Part model, mm, in its own coordinate system. Give positions to 0.01 mm unless a question says otherwise; leave off trailing zeros. Write each loop counter-clockwise with the first axis right and the second up, starting at its lowest first coordinate (ties: lowest second). Pieces come first, ordered by that corner, then holes. Notation, with made-up numbers: (-27.75, -7.5) - (-11.75, -7.5) arc R26 ccw to (-11.75, 10.5) - close; hole circle Ø4 at (53.25, 64.5). An arc over 180 degrees is marked (long way). Answer in a Markdown table with one row per item. Add a question column.
1. Probe line 1 along X through (y, z) = (0.7, -38.1) (3 decimals); line 2 along Z through (x, y) = (28, 0.1); line 3 along Z through (x, y) = (59.5, 1). List the from-to ranges inside material, lowest first.
2. Band-saw the part on A-A on x = 57.15. Write the cut outline in (y, z) (3 decimals).
3. Band-saw the part on B-B on z = -38.1. Write the cut outline in (x, y) (3 decimals).
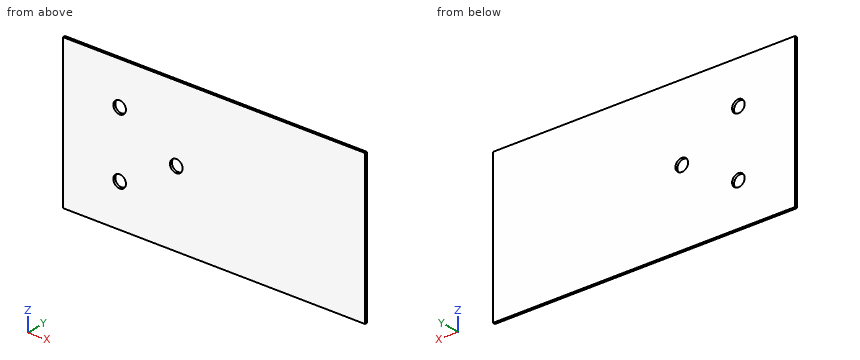
```python
from build123d import *

# Parameters (mm, degrees)
SKETCH2_W                   = 152.4
SKETCH2_H                   = 76.2
BASE_FLANGE1_DEPTH          = 1.2192
F_1_4_0_25_DIAMETER_HOLE1_D = 6.35
CIRPATTERN1_COUNT           = 3


# Sheet-metal steps are written as plain solids
with BuildPart() as part:
    # Sketch2 → Base-Flange1 (new body)
    with BuildSketch(Plane(origin=(0, 0, 0), x_dir=(1, 0, 0), z_dir=(0, 1, 0))):
        with Locations((76.2, 38.1)):
            Rectangle(SKETCH2_W, SKETCH2_H)
    extrude(amount=BASE_FLANGE1_DEPTH)

    # 1/4 (0.25) Diameter Hole1 (through all)
    with Locations(Plane(origin=(57.15, 1.2192, -38.1), x_dir=(0, 0, 1), z_dir=(0, 1, 0))):
        with Locations((0, 0)):
            f_1_4_0_25_diameter_hole1 = Hole(F_1_4_0_25_DIAMETER_HOLE1_D / 2)

    # CirPattern1: 1/4 (0.25) Diameter Hole1 ×3 about axis
    cirpattern1_axis = Axis((38.1, 0, -38.1), (0, 1, 0))
    for i in range(1, CIRPATTERN1_COUNT):
        add(f_1_4_0_25_diameter_hole1.rotate(cirpattern1_axis, i * 360 / CIRPATTERN1_COUNT), mode=Mode.SUBTRACT)


solid = part.part
```
Values:
| question | item | result |
|---|---|---|
| 1 | line 1 | x = 0 to 53.975, 60.325 to 152.4 |
| 1 | line 2 | z = -76.2 to -57.72, -51.48 to -24.72, -18.48 to 0 |
| 1 | line 3 | z = -76.2 to -40.23, -35.97 to 0 |
| 2 | outline | (0, -76.2) - (1.219, -76.2) - (1.219, -41.275) - (0, -41.275) - close; (0, -34.925) - (1.219, -34.925) - (1.219, 0) - (0, 0) - close |
| 3 | outline | (0, 0) - (53.975, 0) - (53.975, 1.219) - (0, 1.219) - close; (60.325, 0) - (152.4, 0) - (152.4, 1.219) - (60.325, 1.219) - close |
